from build123d import *

# Parameters (mm, degrees)
SKETCH1_R           = 3.5
BOSS_EXTRUDE1_DEPTH = 5
SKETCH2_W           = 20
SKETCH2_H           = 3
BOSS_EXTRUDE2_DEPTH = 20


with BuildPart() as part:
    # Sketch1 → Boss-Extrude1 (new body)
    with BuildSketch(Plane(origin=(0, 0, 0), x_dir=(1, 0, 0), z_dir=(0, 1, 0))):
        with BuildLine():
            Line((-46.754410697, 33), (48.5, 33))
            Line((48.5, 33), (60.984651798, 31.862682764))
            ThreePointArc((60.984651798, 31.862682764), (63.227835275, 27.240115524), (66.269368613, 31.381259683))
            Line((66.269368613, 31.381259683), (73.34328665, 30.736845322))
            ThreePointArc((73.34328665, 30.736845322), (78.505606793, 26.614733634), (76.749984847, 20.246127381))
            Line((76.749984847, 20.246127381), (46.754410697, -6))
            Line((46.754410697, -6), (39.754410697, -6))
            Line((39.754410697, -6), (39.754410697, -14))
            Line((39.754410697, -14), (19.754410697, -14))
            Line((19.754410697, -14), (19.754410697, -6))
            Line((19.754410697, -6), (-20.245589303, -6))
            Line((-20.245589303, -6), (-20.245589303, -14))
            Line((-20.245589303, -14), (-40.245589303, -14))
            Line((-40.245589303, -14), (-40.245589303, -6))
            Line((-40.245589303, -6), (-48.5, -6))
            Line((-48.5, -6), (-60.984651798, -4.862682764))
            ThreePointArc((-60.984651798, -4.862682764), (-63.227835275, -0.240115524), (-66.269368613, -4.381259683))
            Line((-66.269368613, -4.381259683), (-73.34328665, -3.736845322))
            ThreePointArc((-73.34328665, -3.736845322), (-78.505606793, 0.385266366), (-76.749984847, 6.753872619))
            Line((-76.749984847, 6.753872619), (-46.754410697, 33))
        make_face()
        with Locations((72.798957199, 24.76158755)):
            Circle(SKETCH1_R, mode=Mode.SUBTRACT)
        with Locations((-72.798957199, 2.23841245)):
            Circle(SKETCH1_R, mode=Mode.SUBTRACT)
        Polygon((-44.5, 27), (52.5, 27), (52.5, 7), (44.5, 0), (-52.5, 0), (-52.5, 20), align=None, mode=Mode.SUBTRACT)
        Polygon((58.5, 21.65), (58.5, 12.25), (68.283497031, 20.810559902), align=None, mode=Mode.SUBTRACT)
        Polygon((-58.5, 14.75), (-68.283497031, 6.189440098), (-58.5, 5.35), align=None, mode=Mode.SUBTRACT)
    extrude(amount=BOSS_EXTRUDE1_DEPTH)

    # Sketch2 → Boss-Extrude2 (add)
    with BuildSketch(Plane.XZ):
        with Locations((-30.245589303, 12.5)):
            Rectangle(SKETCH2_W, SKETCH2_H)
        with Locations((29.754410697, 12.5)):
            Rectangle(SKETCH2_W, SKETCH2_H)
    extrude(amount=BOSS_EXTRUDE2_DEPTH)


solid = part.part
Can you work these out from the model? Positions are in its coordinate system, mm. A direction names the side the tool comes from. Give positions to 0.01 mm unless a question says otherwise; leave off trailing zeros. Loops run counter-clockwise (first coordinate to the right, second up) from the corner with the lowest first, then second, coordinate; pieces in that order, holes last. Notation, with made-up numbers: (33, 62) - (53, 62) arc R22 ccw to (53, 89) - close; hole circle Ø8 at (-10, 76.5). An arc over 180 degrees is marked (long way). One line per item, written item: value.
(1) On a 3-axis mill with a long thin cutter (end or side, diameter ignored), from which of +Z, -Z, +X, -X, +Y, -Y can I reach the whole of each face in a straight line? I mean faces 4 (the face through (0.4, 0, -27.4)), 5 (the face through (39.754, -5, 12)), 6 (the face through (-48.56, 2.46, -23.45)). Say none if no direction works.
Verdict:
face 4: -Z, +X, -X, -Y
face 5: +Z, +X, +Y, -Y
face 6: +Y, -Y
(2) If we section it at C-C, the plane x = 27.5: List the corners of the cut face in (y, z) for me.
Verdict:
outline: (-20, 11) - (0, 11) - (0, 0) - (5, 0) - (5, 14) - (-20, 14) - close; (0, -33) - (5, -33) - (5, -27) - (0, -27) - close
(3) If we section it at B-B, the plane y = -2: List the corners of the cut face in (x, z) for me.
Verdict:
outline: (-40.25, 11) - (-20.25, 11) - (-20.25, 14) - (-40.25, 14) - close; (19.75, 11) - (39.75, 11) - (39.75, 14) - (19.75, 14) - close
(4) I need wall thicknesses on line 1 along X through (y, z) = (0.75, -12); line 2 along X through (y, z) = (3.25, 9); line 3 along Z through (x, y) = (34.5, 2.5). Which ranges of each line are inside material? Lowest first, please.
Verdict:
line 1: -70.75 to -61.64, -58.5 to -52.5, 52.5 to 67.33
line 2: -40.25 to -20.25, 19.75 to 39.75
line 3: -33 to -27, 0 to 14
(5) If we section it at A-A, the plane x = 5.5: List the corners of the cut face in (y, z) for me.
Verdict:
outline: (0, -33) - (5, -33) - (5, -27) - (0, -27) - close; (0, 0) - (5, 0) - (5, 6) - (0, 6) - close
(6) If we mould it in two halves opening along Z, with no side actions, what happens to faces 1 (the face through (30, -10, 11)), 2 (the face through (-20.246, -5, 12)), 3 (the face through (-69.566, 2.465, -0.898))? For each: released by +Z, released by -Z, zero draft, split by the parting line, or undercut.
Verdict:
face 1: released by -Z
face 2: zero draft
face 3: undercut
(7) I'm going to push flat-ended pins straight in: pin 1 (2.5 mm diameter, centred on x = 19, y = 2, fed in from +Z); pin 2 (6 mm diameter, centred on x = -15, z = -2, fed in from -Y); pin 3 (2.5 mm diameter, centred on x = 43, y = 3.5, fed in from +Z); pin 4 (5.5 mm diameter, centred on y = 2, z = -15, fed in from +X). Where does each tip first touch, or does it pass through?
Verdict:
pin 1: z = 14
pin 2: y = 0
pin 3: z = 6
pin 4: x = 73.9
